For this review, take the finished solid that the model builds, in its own axes (mm). Coordinates: 2 decimals unless noted, no trailing zeros. Order: outer loops, then holes, each group sorted by start corner. A loop starts at its lowest first (then second) coordinate and runs counter-clockwise, first axis right, second up.
from build123d import *

# Parameters (mm, degrees)
ESQUISSE2_R             = 1.5
BOSS_EXTRU_1_DEPTH      = 2
ENL_V_MAT_EXTRU_1_REACH = 37.412
ESQUISSE3_R             = 0.5
ESQUISSE4_W             = 9.1
ESQUISSE4_H             = 9.1
BOSS_EXTRU_2_DEPTH      = 1.5
ENL_V_MAT_EXTRU_2_REACH = 37.412
ESQUISSE5_R             = 0.4


with BuildPart() as part:
    # Esquisse2 → Boss.-Extru.1 (new body)
    with BuildSketch(Plane(origin=(0, 0, 0), x_dir=(1, 0, 0), z_dir=(0, 1, 0))):
        with BuildLine():
            Line((0, -3), (22, -3))
            ThreePointArc((22, -3), (24.121320344, -2.121320344), (25, 0))
            Line((25, 0), (25, 22))
            ThreePointArc((25, 22), (24.121320344, 24.121320344), (22, 25))
            Line((22, 25), (0, 25))
            ThreePointArc((0, 25), (-2.121320344, 24.121320344), (-3, 22))
            Line((-3, 22), (-3, 0))
            ThreePointArc((-3, 0), (-2.121320344, -2.121320344), (0, -3))
        make_face()
        with Locations(Location((0, 0, 0), (0, 0, 270))):
            Circle(ESQUISSE2_R, mode=Mode.SUBTRACT)
        with Locations(Location((22, 22, 0), (0, 0, 270))):
            Circle(ESQUISSE2_R, mode=Mode.SUBTRACT)
    extrude(amount=BOSS_EXTRU_1_DEPTH)

    # Esquisse3 → Enlèv. mat.-Extru.1 (cut, up to next)
    with BuildSketch(Plane(origin=(0, 2, 0), x_dir=(1, 0, 0), z_dir=(0, 1, 0)), mode=Mode.PRIVATE) as enl_v_mat_extru_1_sk1:
        with Locations(Location((5.94, 17.9, 0), (0, 0, 270))):
            Circle(ESQUISSE3_R)
    enl_v_mat_extru_1_tool1 = extrude(enl_v_mat_extru_1_sk1.sketch, amount=-ENL_V_MAT_EXTRU_1_REACH, mode=Mode.PRIVATE) & part.part
    # Esquisse3 → Enlèv. mat.-Extru.1 (cut, up to next)
    with BuildSketch(Plane(origin=(0, 2, 0), x_dir=(1, 0, 0), z_dir=(0, 1, 0)), mode=Mode.PRIVATE) as enl_v_mat_extru_1_sk2:
        with Locations(Location((8.48, 17.9, 0), (0, 0, 270))):
            Circle(ESQUISSE3_R)
    enl_v_mat_extru_1_tool2 = extrude(enl_v_mat_extru_1_sk2.sketch, amount=-ENL_V_MAT_EXTRU_1_REACH, mode=Mode.PRIVATE) & part.part
    # Esquisse3 → Enlèv. mat.-Extru.1 (cut, up to next)
    with BuildSketch(Plane(origin=(0, 2, 0), x_dir=(1, 0, 0), z_dir=(0, 1, 0)), mode=Mode.PRIVATE) as enl_v_mat_extru_1_sk3:
        with Locations(Location((11.02, 17.9, 0), (0, 0, 270))):
            Circle(ESQUISSE3_R)
    enl_v_mat_extru_1_tool3 = extrude(enl_v_mat_extru_1_sk3.sketch, amount=-ENL_V_MAT_EXTRU_1_REACH, mode=Mode.PRIVATE) & part.part
    # Esquisse3 → Enlèv. mat.-Extru.1 (cut, up to next)
    with BuildSketch(Plane(origin=(0, 2, 0), x_dir=(1, 0, 0), z_dir=(0, 1, 0)), mode=Mode.PRIVATE) as enl_v_mat_extru_1_sk4:
        with Locations(Location((13.56, 17.9, 0), (0, 0, 270))):
            Circle(ESQUISSE3_R)
    enl_v_mat_extru_1_tool4 = extrude(enl_v_mat_extru_1_sk4.sketch, amount=-ENL_V_MAT_EXTRU_1_REACH, mode=Mode.PRIVATE) & part.part
    # Esquisse3 → Enlèv. mat.-Extru.1 (cut, up to next)
    with BuildSketch(Plane(origin=(0, 2, 0), x_dir=(1, 0, 0), z_dir=(0, 1, 0)), mode=Mode.PRIVATE) as enl_v_mat_extru_1_sk5:
        with Locations(Location((16.1, 17.9, 0), (0, 0, 270))):
            Circle(ESQUISSE3_R)
    enl_v_mat_extru_1_tool5 = extrude(enl_v_mat_extru_1_sk5.sketch, amount=-ENL_V_MAT_EXTRU_1_REACH, mode=Mode.PRIVATE) & part.part
    # Esquisse3 → Enlèv. mat.-Extru.1 (cut, up to next)
    with BuildSketch(Plane(origin=(0, 2, 0), x_dir=(1, 0, 0), z_dir=(0, 1, 0)), mode=Mode.PRIVATE) as enl_v_mat_extru_1_sk6:
        with Locations(Location((3.4, 17.9, 0), (0, 0, 270))):
            Circle(ESQUISSE3_R)
    enl_v_mat_extru_1_tool6 = extrude(enl_v_mat_extru_1_sk6.sketch, amount=-ENL_V_MAT_EXTRU_1_REACH, mode=Mode.PRIVATE) & part.part
    add(enl_v_mat_extru_1_tool1.solids().sort_by_distance((5.94, 2, -17.9))[0], mode=Mode.SUBTRACT)
    add(enl_v_mat_extru_1_tool2.solids().sort_by_distance((8.48, 2, -17.9))[0], mode=Mode.SUBTRACT)
    add(enl_v_mat_extru_1_tool3.solids().sort_by_distance((11.02, 2, -17.9))[0], mode=Mode.SUBTRACT)
    add(enl_v_mat_extru_1_tool4.solids().sort_by_distance((13.56, 2, -17.9))[0], mode=Mode.SUBTRACT)
    add(enl_v_mat_extru_1_tool5.solids().sort_by_distance((16.1, 2, -17.9))[0], mode=Mode.SUBTRACT)
    add(enl_v_mat_extru_1_tool6.solids().sort_by_distance((3.4, 2, -17.9))[0], mode=Mode.SUBTRACT)

    # Esquisse4 → Boss.-Extru.2 (add)
    with BuildSketch(Plane(origin=(0, 2, 0), x_dir=(1, 0, 0), z_dir=(0, 1, 0))):
        with Locations((7.2, 7.8)):
            Rectangle(ESQUISSE4_W, ESQUISSE4_H)
    extrude(amount=BOSS_EXTRU_2_DEPTH)

    # Esquisse5 → Enlèv. mat.-Extru.2 (cut, up to next)
    with BuildSketch(Plane(origin=(0, 2, 0), x_dir=(1, 0, 0), z_dir=(0, 1, 0)), mode=Mode.PRIVATE) as enl_v_mat_extru_2_sk1:
        with Locations(Location((17.98, 1.44, 0), (0, 0, 270))):
            Circle(ESQUISSE5_R)
    enl_v_mat_extru_2_tool1 = extrude(enl_v_mat_extru_2_sk1.sketch, amount=-ENL_V_MAT_EXTRU_2_REACH, mode=Mode.PRIVATE) & part.part
    # Esquisse5 → Enlèv. mat.-Extru.2 (cut, up to next)
    with BuildSketch(Plane(origin=(0, 2, 0), x_dir=(1, 0, 0), z_dir=(0, 1, 0)), mode=Mode.PRIVATE) as enl_v_mat_extru_2_sk2:
        with Locations(Location((17.98, 3.98, 0), (0, 0, 270))):
            Circle(ESQUISSE5_R)
    enl_v_mat_extru_2_tool2 = extrude(enl_v_mat_extru_2_sk2.sketch, amount=-ENL_V_MAT_EXTRU_2_REACH, mode=Mode.PRIVATE) & part.part
    # Esquisse5 → Enlèv. mat.-Extru.2 (cut, up to next)
    with BuildSketch(Plane(origin=(0, 2, 0), x_dir=(1, 0, 0), z_dir=(0, 1, 0)), mode=Mode.PRIVATE) as enl_v_mat_extru_2_sk3:
        with Locations(Location((17.98, 6.52, 0), (0, 0, 270))):
            Circle(ESQUISSE5_R)
    enl_v_mat_extru_2_tool3 = extrude(enl_v_mat_extru_2_sk3.sketch, amount=-ENL_V_MAT_EXTRU_2_REACH, mode=Mode.PRIVATE) & part.part
    add(enl_v_mat_extru_2_tool1.solids().sort_by_distance((17.98, 2, -1.44))[0], mode=Mode.SUBTRACT)
    add(enl_v_mat_extru_2_tool2.solids().sort_by_distance((17.98, 2, -3.98))[0], mode=Mode.SUBTRACT)
    add(enl_v_mat_extru_2_tool3.solids().sort_by_distance((17.98, 2, -6.52))[0], mode=Mode.SUBTRACT)


solid = part.part
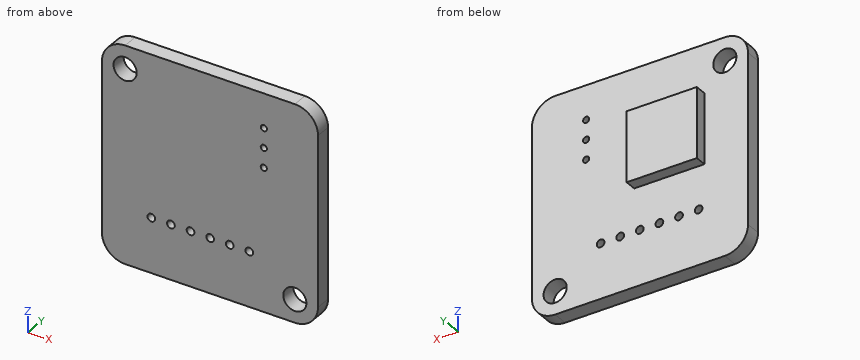
1. Take a section at A-A, the plane x = 16.1. Give the boundary of the cut face in (y, z).
Answer below:
outline: (0, -25) - (2, -25) - (2, -18.4) - (0, -18.4) - close; (0, -17.4) - (2, -17.4) - (2, 3) - (0, 3) - close
2. Take a section at B-B, the plane z = -6.52. Give the boundary of the cut face in (x, y).
Answer below:
outline: (-3, 0) - (17.58, 0) - (17.58, 2) - (11.75, 2) - (11.75, 3.5) - (2.65, 3.5) - (2.65, 2) - (-3, 2) - close; (18.38, 0) - (25, 0) - (25, 2) - (18.38, 2) - close
3. To check wall thickness, follow L1, parallel to Z at x = 17.98, y = 1.25; L2, parallel to X at y = 0.55, z = -6.52; L3, parallel to Y at x = 1.25, z = -19.75. State the ranges of each line that lie inside material, in increasing order.
Answer below:
L1: z = -25 to -6.92, -6.12 to -4.38, -3.58 to -1.84, -1.04 to 3
L2: x = -3 to 17.58, 18.38 to 25
L3: y = 0 to 2
4. Take a section at C-C, the plane y = 0.8. Give the number of separate pieces and of enclosed holes in the cut face, plus the area to 3 significant figures.
Answer below:
separate pieces: 1
enclosed holes: 11
area: 756 mm2
5. Take a section at D-D, the plane x = 11.02. Give the boundary of the cut face in (y, z), plus the area to 4 significant figures.
Answer below:
outline: (0, -25) - (2, -25) - (2, -18.4) - (0, -18.4) - close; (0, -17.4) - (2, -17.4) - (2, -12.35) - (3.5, -12.35) - (3.5, -3.25) - (2, -3.25) - (2, 3) - (0, 3) - close
area: 67.65 mm2
6. Clearance check with flat-ended pins moving along their axes: pin 1 Ø0.8 at (x, y) = (8.5, 3) entering from +Z; pin 2 Ø0.8 at (x, y) = (8, 2.5) entering from -Z; pin 3 Ø1.2 at (y, z) = (3, -6) entering from -X. State where each tip first meets the part, or that it passes through.
Answer below:
pin 1: stops at z = -3.25
pin 2: stops at z = -12.35
pin 3: stops at x = 2.65
